from build123d import *

# Parameters (mm, degrees)
SKETCH1_W               = 1500
SKETCH1_H               = 500
BOSS_EXTRUDE1_DEPTH     = 80
FILLET2_R               = 10
CUT_EXTRUDE2_START      = 80
SKETCH7_W               = 720
SKETCH7_H               = 439.016917436
CUT_EXTRUDE2_DEPTH      = 2
CUT_EXTRUDE1_START      = 78
SKETCH5_W               = 66
SKETCH5_H               = 45
CUT_EXTRUDE1_DEPTH      = 10
CUT_EXTRUDE3_START      = 80
SKETCH8_R               = 5
CUT_EXTRUDE3_DEPTH      = 875.606821013
CUT_EXTRUDE4_DEPTH      = 100
CUT_EXTRUDE4_DEPTH_BACK = 100
SKETCH9_W               = 1310.383503898
SKETCH9_H               = 40
BOSS_EXTRUDE2_START     = 40
SKETCH10_W              = 50
SKETCH10_H              = 200
BOSS_EXTRUDE2_DEPTH     = 40


with BuildPart() as part:
    # Sketch1 → Boss-Extrude1 (new body)
    with BuildSketch(Plane(origin=(0, 0, 0), x_dir=(1, 0, 0), z_dir=(0, 1, 0))):
        Rectangle(SKETCH1_W, SKETCH1_H)
    extrude(amount=BOSS_EXTRUDE1_DEPTH)

    # Fillet2
    fillet2_edges = [part.edges().sort_by_distance(p)[0] for p in [
        (-750, 80, 0),
        (0, 80, 250),
        (750, 80, 0),
        (0, 80, -250),
    ]]
    fillet(fillet2_edges, radius=FILLET2_R)

    # Sketch7 → Cut-Extrude2 (cut)
    with BuildSketch(Plane(origin=(0, 0, 0), x_dir=(1, 0, 0), z_dir=(0, 1, 0)).offset(CUT_EXTRUDE2_START)):
        with Locations((0, 157.008458718)):
            Rectangle(SKETCH7_W, SKETCH7_H)
    extrude(amount=-CUT_EXTRUDE2_DEPTH, mode=Mode.SUBTRACT)

    # Sketch5 → Cut-Extrude1 (cut)
    with BuildSketch(Plane(origin=(0, 0, 0), x_dir=(1, 0, 0), z_dir=(0, 1, 0)).offset(CUT_EXTRUDE1_START)):
        with BuildLine():
            Line((-340, 52.5), (340, 52.5))
            ThreePointArc((340, 52.5), (347.071067812, 49.571067812), (350, 42.5))
            Line((350, 42.5), (350, -42.5))
            ThreePointArc((350, -42.5), (347.071067812, -49.571067812), (340, -52.5))
            Line((340, -52.5), (-340, -52.5))
            ThreePointArc((-340, -52.5), (-347.071067812, -49.571067812), (-350, -42.5))
            Line((-350, -42.5), (-350, 42.5))
            ThreePointArc((-350, 42.5), (-347.071067812, 49.571067812), (-340, 52.5))
        make_face()
        with BuildLine():
            Line((-340, 47.5), (-279, 47.5))
            Line((-279, 47.5), (-279, 7.071067812))
            ThreePointArc((-279, 7.071067812), (-281.803300859, 5.303300859), (-283.571067812, 2.5))
            Line((-283.571067812, 2.5), (-345, 2.5))
            Line((-345, 2.5), (-345, 42.5))
            ThreePointArc((-345, 42.5), (-343.535533906, 46.035533906), (-340, 47.5))
        make_face(mode=Mode.SUBTRACT)
        with BuildLine():
            Line((-340, -47.5), (-279, -47.5))
            Line((-279, -47.5), (-279, -7.071067812))
            ThreePointArc((-279, -7.071067812), (-281.803300859, -5.303300859), (-283.571067812, -2.5))
            Line((-283.571067812, -2.5), (-345, -2.5))
            Line((-345, -2.5), (-345, -42.5))
            ThreePointArc((-345, -42.5), (-343.535533906, -46.035533906), (-340, -47.5))
        make_face(mode=Mode.SUBTRACT)
        with BuildLine():
            Line((345, 42.5), (345, 2.5))
            Line((345, 2.5), (293.571067812, 2.5))
            ThreePointArc((293.571067812, 2.5), (291.803300859, 5.303300859), (289, 7.071067812))
            Line((289, 7.071067812), (289, 47.5))
            Line((289, 47.5), (340, 47.5))
            ThreePointArc((340, 47.5), (343.535533906, 46.035533906), (345, 42.5))
        make_face(mode=Mode.SUBTRACT)
        with Locations((-175, -25)):
            Rectangle(SKETCH5_W, SKETCH5_H, mode=Mode.SUBTRACT)
        with BuildLine():
            Line((0, 47.5), (0, 7.071067812))
            ThreePointArc((0, 7.071067812), (-2.803300859, 5.303300859), (-4.571067812, 2.5))
            Line((-4.571067812, 2.5), (-66, 2.5))
            Line((-66, 2.5), (-66, 47.5))
            Line((-66, 47.5), (0, 47.5))
        make_face(mode=Mode.SUBTRACT)
        with BuildLine():
            Line((5, 47.5), (5, 7.071067812))
            ThreePointArc((5, 7.071067812), (7.803300859, 5.303300859), (9.571067812, 2.5))
            Line((9.571067812, 2.5), (71, 2.5))
            Line((71, 2.5), (71, 47.5))
            Line((71, 47.5), (5, 47.5))
        make_face(mode=Mode.SUBTRACT)
        with Locations((-104, 25)):
            Rectangle(SKETCH5_W, SKETCH5_H, mode=Mode.SUBTRACT)
        with Locations((109, 25)):
            Rectangle(SKETCH5_W, SKETCH5_H, mode=Mode.SUBTRACT)
        with Locations((180, 25)):
            Rectangle(SKETCH5_W, SKETCH5_H, mode=Mode.SUBTRACT)
        with BuildLine():
            Line((218, 47.5), (218, 2.5))
            Line((218, 2.5), (279.428932188, 2.5))
            ThreePointArc((279.428932188, 2.5), (281.196699141, 5.303300859), (284, 7.071067812))
            Line((284, 7.071067812), (284, 47.5))
            Line((284, 47.5), (218, 47.5))
        make_face(mode=Mode.SUBTRACT)
        with Locations((-175, 25)):
            Rectangle(SKETCH5_W, SKETCH5_H, mode=Mode.SUBTRACT)
        with BuildLine():
            Line((-213, 47.5), (-213, 2.5))
            Line((-213, 2.5), (-269.428932188, 2.5))
            ThreePointArc((-269.428932188, 2.5), (-271.196699141, 5.303300859), (-274, 7.071067812))
            Line((-274, 7.071067812), (-274, 47.5))
            Line((-274, 47.5), (-213, 47.5))
        make_face(mode=Mode.SUBTRACT)
        with BuildLine():
            Line((-274, -7.071067812), (-274, -47.5))
            Line((-274, -47.5), (-213, -47.5))
            Line((-213, -47.5), (-213, -2.5))
            Line((-213, -2.5), (-269.428932188, -2.5))
            ThreePointArc((-269.428932188, -2.5), (-271.196699141, -5.303300859), (-274, -7.071067812))
        make_face(mode=Mode.SUBTRACT)
        with Locations((-104, -25)):
            Rectangle(SKETCH5_W, SKETCH5_H, mode=Mode.SUBTRACT)
        with BuildLine():
            Line((-66, -2.5), (-4.571067812, -2.5))
            ThreePointArc((-4.571067812, -2.5), (-2.803300859, -5.303300859), (0, -7.071067812))
            Line((0, -7.071067812), (0, -47.5))
            Line((0, -47.5), (-66, -47.5))
            Line((-66, -47.5), (-66, -2.5))
        make_face(mode=Mode.SUBTRACT)
        with BuildLine():
            Line((5, -7.071067812), (5, -47.5))
            Line((5, -47.5), (71, -47.5))
            Line((71, -47.5), (71, -2.5))
            Line((71, -2.5), (9.571067812, -2.5))
            ThreePointArc((9.571067812, -2.5), (7.803300859, -5.303300859), (5, -7.071067812))
        make_face(mode=Mode.SUBTRACT)
        with Locations((109, -25)):
            Rectangle(SKETCH5_W, SKETCH5_H, mode=Mode.SUBTRACT)
        with Locations((180, -25)):
            Rectangle(SKETCH5_W, SKETCH5_H, mode=Mode.SUBTRACT)
        with BuildLine():
            Line((218, -2.5), (218, -47.5))
            Line((218, -47.5), (284, -47.5))
            Line((284, -47.5), (284, -7.071067812))
            ThreePointArc((284, -7.071067812), (281.196699141, -5.303300859), (279.428932188, -2.5))
            Line((279.428932188, -2.5), (218, -2.5))
        make_face(mode=Mode.SUBTRACT)
        with BuildLine():
            Line((289, -7.071067812), (289, -47.5))
            Line((289, -47.5), (340, -47.5))
            ThreePointArc((340, -47.5), (343.535533906, -46.035533906), (345, -42.5))
            Line((345, -42.5), (345, -2.5))
            Line((345, -2.5), (293.571067812, -2.5))
            ThreePointArc((293.571067812, -2.5), (291.803300859, -5.303300859), (289, -7.071067812))
        make_face(mode=Mode.SUBTRACT)
    extrude(amount=-CUT_EXTRUDE1_DEPTH, mode=Mode.SUBTRACT)

    # Sketch8 → Cut-Extrude3 (cut, through all)
    with BuildSketch(Plane(origin=(0, 0, 0), x_dir=(1, 0, 0), z_dir=(0, 1, 0)).offset(CUT_EXTRUDE3_START)):
        with Locations(Location((-276.5, 0, 0), (0, 0, 270))):
            Circle(SKETCH8_R)
        with Locations(Location((2.5, 0, 0), (0, 0, 270))):
            Circle(SKETCH8_R)
        with Locations(Location((286.5, 0, 0), (0, 0, 270))):
            Circle(SKETCH8_R)
    extrude(amount=-CUT_EXTRUDE3_DEPTH, mode=Mode.SUBTRACT)

    # Sketch9 → Cut-Extrude4 (cut, two sides: drawn at the far end of the back side and taken through both)
    with BuildSketch(Plane.XY.offset(-CUT_EXTRUDE4_DEPTH_BACK)):
        with Locations((-274.195529116, 20)):
            Rectangle(SKETCH9_W, SKETCH9_H)
    extrude(amount=CUT_EXTRUDE4_DEPTH + CUT_EXTRUDE4_DEPTH_BACK, mode=Mode.SUBTRACT)

    # Sketch10 → Boss-Extrude2 (add)
    with BuildSketch(Plane(origin=(0, 0, 0), x_dir=(1, 0, 0), z_dir=(0, 1, 0)).offset(BOSS_EXTRUDE2_START)):
        with Locations((-137, 0)):
            Rectangle(SKETCH10_W, SKETCH10_H)
        with Locations((144.5, 0)):
            Rectangle(SKETCH10_W, SKETCH10_H)
        with Locations((-416, 0)):
            Rectangle(SKETCH10_W, SKETCH10_H)
    extrude(amount=-BOSS_EXTRUDE2_DEPTH)


solid = part.part
Verification items for the finished model (mm, model axes). A direction names the side the tool comes from. Coordinates: 2 decimals unless noted, no trailing zeros. Write each loop counter-clockwise with the first axis right and the second up, starting at its lowest first coordinate (ties: lowest second). Pieces come first, ordered by that corner, then holes. Notation, with made-up numbers: M -37.5,-21 L -22.5,-21 A13 ccw -22.5,0 Z; hole C -3,65 d1. An arc over 180 degrees is marked long. Use CSV: the item, a comma, the result in double quotes.
Q1. Set-up check for faces 1 (the flat face through (750, 35, 3)), 2 (the flat face through (-391, 20, 1)), 3 (the flat face through (28, 68, 0)), 4 (the flat face through (317, 78, 25)), 5 (the flat face through (156, 0, -4)): record each of +Z, -Z, +X, -X, +Y, -Y from which the full face is reachable in a straight line by a thin tool's end or side.
Computed values:
face 1,"+Z, -Z, +X, +Y, -Y"
face 2,"-Y"
face 3,"+Y"
face 4,"-Z, +Y"
face 5,"+Z, -Z, +X, -X, -Y"
Q2. Section check A-A, the plane y = 18.5. Enter the section's corners in (x, z), and give its area (3 significant figures).
Computed values:
outline,"M -750,-250 L 750,-250 L 750,250 L -750,250 L -750,100 L -441,100 L -441,-100 L -750,-100 Z; hole M -391,-100 L -162,-100 L -162,100 L -391,100 Z; hole M -112,-100 L 119.5,-100 L 119.5,100 L -112,100 Z; hole M 169.5,-100 L 381,-100 L 381,100 L 169.5,100 Z"
area,"554,000 mm²"
Q3. Go/stop test with flat-tipped pins: P1, Ø5, axis at x = 310.5, y = 74.5, coming from the +Z side; P2, Ø22.5, axis at x = -170, z = -17, coming from the +Y side; P3, Ø8, axis at y = 75, z = -30.5, coming from the -X side. Record where each tip stops, or that it passes through.
Computed values:
P1,"z = 249.8"
P2,"y = 78"
P3,"x = -749.95"
Q4. Mould release check, pull along Z, two halves, no side actions. Record for faces 6 (the flat face through (-10, 35, 250)), 7 (the flat face through (380.996, 20, -1)), 8 (the flat face through (-175, 78, 25)): pulls with the +Z half, pulls with the -Z half, needs draft (parallel to the pull), parting line crosses it, or undercut.
Computed values:
face 6,"pulls with the +Z half"
face 7,"undercut"
face 8,"needs draft"
Q5. Thickness scan on line 1 along X through (y, z) = (39.5, -92); line 2 along Z through (x, y) = (-276.5, 62.25); line 3 along Z through (x, y) = (-599, 22.5). Record the ranges inside material, lowest first. Write a range as [from, to].
Computed values:
line 1,"[-441, -391], [-162, -112], [119.5, 169.5], [381, 750]"
line 2,"[-250, -5], [5, 250]"
line 3,"[-250, -100], [100, 250]"
Q6. Section check C-C, the plane x = -46. Enter the section's corners in (y, z), and give its area (3 significant figures).
Computed values:
outline,"M 0,-250 L 70,-250 A10 ccw 78,-246 L 78,-52.5 L 68,-52.5 L 68,-47.5 L 78,-47.5 L 78,-2.5 L 68,-2.5 L 68,2.5 L 78,2.5 L 78,47.5 L 68,47.5 L 68,52.5 L 78,52.5 L 78,62.5 L 80,62.5 L 80,240 A10 ccw 70,250 L 0,250 L 0,100 L 40,100 L 40,-100 L 0,-100 Z"
area,"31,200 mm²"
Q7. Section check B-B, the plane z = -68.5. Enter the section's corners in (x, y).
Computed values:
outline,"M -750,40 L -441,40 L -441,0 L -391,0 L -391,40 L -162,40 L -162,0 L -112,0 L -112,40 L 119.5,40 L 119.5,0 L 169.5,0 L 169.5,40 L 381,40 L 381,0 L 750,0 L 750,70 A10 ccw 740,80 L 360,80 L 360,78 L -360,78 L -360,80 L -740,80 A10 ccw -750,70 Z"
